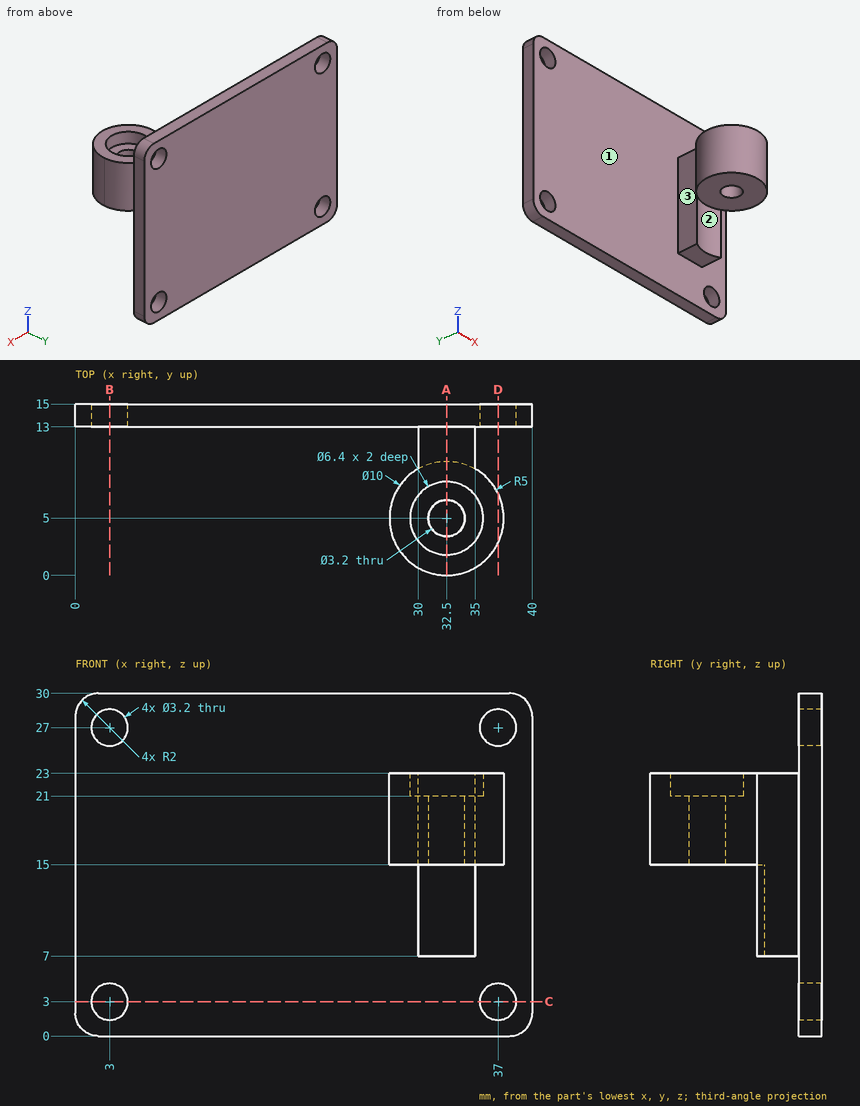
Input: dimensioned drawing with shaded views. Units: mm. Origin: part minimum x, y, z. Round coordinates to 2 decimals unless told otherwise and drop trailing zeros. Loops run counter-clockwise (first coordinate to the right, second up) from the corner with the lowest first, then second, coordinate; pieces in that order, holes last. Notation, with made-up numbers: M 62,58.5 L 93,58.5 A14 cw 93,69.5 Z; hole C 89,11.5 d7. An arc over 180 degrees is marked long. One line per question, with ' | ' between items.
(1) Pull-direction query (X, two-part tool) for the marked faces 1, 2 and 3; classes: +X half, -X half, draft (parallel to the pull), parting line (faces both ways), or undercut.
Check result:
face 1: draft | face 2: undercut | face 3: -X half
(2) Material intervals for line 1 along Z through (x, y) = (3, 14.05); line 2 along Y through (x, z) = (32.5, 21.5); line 3 along Y through (x, z) = (10, 20), sorted ascending. Write a range as from..to.
Check result:
line 1: z = 0..1.4, 4.6..25.4, 28.6..30 | line 2: y = 0..1.8, 8.2..15 | line 3: y = 13..15
(3) Contact query for flat-ended pins moving along their axis: P1, Ø1.1, axis at y = 11.5, z = 18, coming from the +X side; P2, Ø3, axis at x = 31, y = 4.5, coming from the +Z side; P3, Ø15, axis at x = 15, z = 11, coming from the -Y side. Output: stop coordinate, or through.
Check result:
P1: stops at x = 35 | P2: stops at z = 21 | P3: stops at y = 13
(4) Cut plane A-A on x = 32.5. Return the cut outline in (y, z), plus the area to 3 significant figures.
Check result:
outline: M 0,15 L 3.4,15 L 3.4,21 L 1.8,21 L 1.8,23 L 0,23 Z; M 6.6,15 L 10,15 L 10,7 L 13,7 L 13,0 L 15,0 L 15,30 L 13,30 L 13,23 L 8.2,23 L 8.2,21 L 6.6,21 Z | area: 156 mm2
(5) Cut plane D-D on x = 37. Return the cut outline in (y, z), plus the area to 3 significant figures.
Check result:
outline: M 2.82,15 L 7.18,15 L 7.18,23 L 2.82,23 Z; M 13,0 L 15,0 L 15,1.4 L 13,1.4 Z; M 13,4.6 L 15,4.6 L 15,25.4 L 13,25.4 Z; M 13,28.6 L 15,28.6 L 15,30 L 13,30 Z | area: 82.1 mm2
(6) Cut plane B-B on x = 3. Return the cut outline in (y, z).
Check result:
outline: M 13,0 L 15,0 L 15,1.4 L 13,1.4 Z; M 13,4.6 L 15,4.6 L 15,25.4 L 13,25.4 Z; M 13,28.6 L 15,28.6 L 15,30 L 13,30 Z
(7) Cut plane C-C on z = 3. Return the cut outline in (x, y).
Check result:
outline: M 0,13 L 1.4,13 L 1.4,15 L 0,15 Z; M 4.6,13 L 35.4,13 L 35.4,15 L 4.6,15 Z; M 38.6,13 L 40,13 L 40,15 L 38.6,15 Z
